Verification items for the finished model (mm, model axes). Face numbers are marked on the shaded views. Coordinates: 2 decimals unless noted, no trailing zeros. Write each loop counter-clockwise with the first axis right and the second up, starting at its lowest first coordinate (ties: lowest second). Pieces come first, ordered by that corner, then holes. Notation, with made-up numbers: (43, 40.25) -> (92, 40.25) arc R12 cw to (92, 52.25) -> close; hole circle Ø9 at (-5.75, 27). An arc over 180 degrees is marked (long way). Write item = value, one per line. Start each with the question number.
(1) Material ranges on probe 1 along Y at (x, z) = (0, -44.05); probe 2 along Y at (x, z) = (0, 43.7); probe 3 along X at (y, z) = (87, -1.5), recorded low to high. Write a range as [from, to].
(2) Section check C-C (y = 30). State how many separate pieces and enclosed holes the cut face has, plus the area to 3 significant figures.
(3) Section check B-B (x = 0). Record the cut outline in (y, z), plus the area to 3 significant figures.
(4) Section check A-A (z = 0). Record the cut outline in (x, y).
(5) Mould release check, pull along Z, two halves, no side actions. Record for the marked faces 1 and 2: released by +Z, released by -Z, zero draft, split by the parting line, or undercut.
(6) Section check D-D (x = -14). Record the cut outline in (y, z).
(7) Gauge pin test, flat ends, axial feed: pin 1 Ø2.5 at (x, z) = (1.5, -43) entering from -Y; pin 2 Ø12 at (y, z) = (53.5, -31.5) entering from -X; pin 3 Ø1.5 at (y, z) = (32.5, 22) entering from +X. Record the tip position at first contact, or that the pin passes through.
```python
from build123d import *

# Parameters (mm, degrees)
SKIZZE1_R                       = 44.5
SKIZZE1_R_2                     = 43
AUFSATZ_LINEAR_AUSTRAGEN1_DEPTH = 120
SKIZZE2_R                       = 4
SCHNITT_LINEAR_AUSTRAGEN1_DEPTH = 45.5
SKIZZE3_R                       = 2
SCHNITT_LINEAR_AUSTRAGEN2_DEPTH = 45.5000001
KREISMUSTER1_COUNT              = 8
SKIZZE4_W                       = 24
SKIZZE4_H                       = 24.318999769
SCHNITT_LINEAR_AUSTRAGEN3_DEPTH = 45.50000012
VERRUNDUNG1_R                   = 2


with BuildPart() as part:
    # Skizze1 → Aufsatz-Linear austragen1 (new body)
    with BuildSketch(Plane(origin=(0, 0, 0), x_dir=(1, 0, 0), z_dir=(0, 1, 0))):
        Circle(SKIZZE1_R)
        Circle(SKIZZE1_R_2, mode=Mode.SUBTRACT)
    extrude(amount=AUFSATZ_LINEAR_AUSTRAGEN1_DEPTH)

    # Skizze2 → Schnitt-Linear austragen1 (cut, through all)
    with BuildSketch(Plane.XY):
        with Locations((0, 50)):
            Circle(SKIZZE2_R)
    extrude(amount=-SCHNITT_LINEAR_AUSTRAGEN1_DEPTH, mode=Mode.SUBTRACT)

    # Skizze3 → Schnitt-Linear austragen2 (cut, through all)
    with BuildSketch(Plane.XY):
        with Locations((0, 30)):
            Circle(SKIZZE3_R)
    schnitt_linear_austragen2 = extrude(amount=-SCHNITT_LINEAR_AUSTRAGEN2_DEPTH, mode=Mode.SUBTRACT)

    # Kreismuster1: Schnitt-Linear austragen2 ×8 about axis
    kreismuster1_axis = Axis((0, 120, 0), (0, -1, 0))
    for i in range(1, KREISMUSTER1_COUNT):
        add(schnitt_linear_austragen2.rotate(kreismuster1_axis, i * 360 / KREISMUSTER1_COUNT), mode=Mode.SUBTRACT)

    # Skizze4 → Schnitt-Linear austragen3 (cut, through all)
    with BuildSketch(Plane.XY):
        with Locations((2, 12.159499885)):
            Rectangle(SKIZZE4_W, SKIZZE4_H)
    extrude(amount=-SCHNITT_LINEAR_AUSTRAGEN3_DEPTH, mode=Mode.SUBTRACT)

    # Verrundung1
    verrundung1_edges = [part.edges().sort_by_distance(p)[0] for p in [
        (-10, 24.318999769, -42.591448462),
        (14, 24.318999769, -41.448743111),
    ]]
    fillet(verrundung1_edges, radius=VERRUNDUNG1_R)


solid = part.part
```
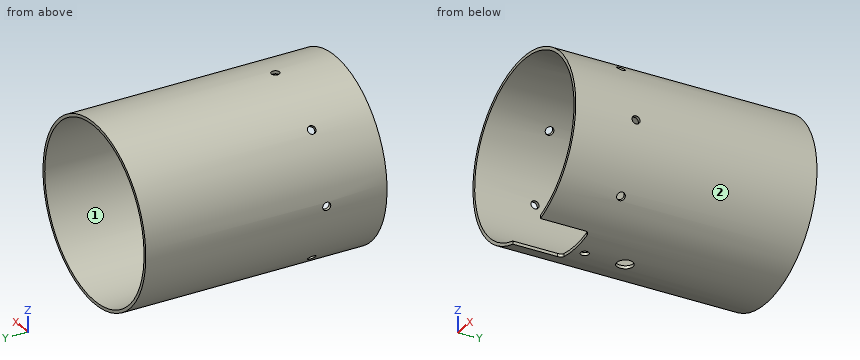
Response:
q1.probe_1 = [24.32, 28], [32, 46], [54, 120]
q1.probe_2 = [0, 28], [32, 120]
q1.probe_3 = [-44.47, -42.97], [42.97, 44.47]
q2.separate_pieces = 8
q2.enclosed_holes = 0
q2.area = 364 mm2
q3.outline = (0, 43) -> (28, 43) -> (28, 44.5) -> (0, 44.5) -> close; (24.32, -44.5) -> (28, -44.5) -> (28, -43) -> (24.32, -43) -> close; (32, -44.5) -> (46, -44.5) -> (46, -43) -> (32, -43) -> close; (32, 43) -> (120, 43) -> (120, 44.5) -> (32, 44.5) -> close; (54, -44.5) -> (120, -44.5) -> (120, -43) -> (54, -43) -> close
q3.area = 300 mm2
q4.outline = (-44.5, 0) -> (-43, 0) -> (-43, 28) -> (-44.5, 28) -> close; (-44.5, 32) -> (-43, 32) -> (-43, 120) -> (-44.5, 120) -> close; (43, 0) -> (44.5, 0) -> (44.5, 28) -> (43, 28) -> close; (43, 32) -> (44.5, 32) -> (44.5, 120) -> (43, 120) -> close
q5.face_1 = undercut
q5.face_2 = split by the parting line
q6.outline = (0, -42.24) -> (120, -42.24) -> (120, -40.66) -> (0, -40.66) -> close; (0, 40.66) -> (120, 40.66) -> (120, 42.24) -> (0, 42.24) -> close
q7.pin_1 = 24.32
q7.pin_2 = -36.47
q7.pin_3 = 39.1
